Geometry: final body of the model. Coordinates: model frame, mm. Face numbers are marked on the shaded views. A direction names the side the tool comes from. Give positions to 0.01 mm unless a question says otherwise; leave off trailing zeros. Write each loop counter-clockwise with the first axis right and the second up, starting at its lowest first coordinate (ties: lowest second). Pieces come first, ordered by that corner, then holes. Notation, with made-up numbers: (49, -35) -> (62, -35) arc R27 cw to (62, 4) -> close; hole circle Ø10 at (24, -2.75). An arc over 180 degrees is marked (long way). Use CSV: the item, a comma, the result in double quotes. Start each with the question number.
1) Material intervals for line 1 (Z direction, x = 0, y = 8); line 2 (X direction, y = -23, z = -2); line 3 (Y direction, x = -23, z = -13), sorted ascending. Write a range as [from, to].
2) Section A-A (y = 4.5). Output: boundary loops of the cut face in (x, z) (3 decimals).
3) Section C-C (y = -8). Output: boundary loops of the cut face in (x, z).
4) Draft query along X for the marked faces 4, 5 and 6. Return one class per face: pulls with the +X half, pulls with the -X half, needs draft (parallel to the pull), parting line crosses it, or undercut.
5) Contact query for flat-ended pins moving along their axis: P1, Ø2, axis at x = -16.5, y = 3, coming from the +Z side; P2, Ø3, axis at x = 22, z = 0, coming from the -Y side; P3, Ø1, axis at x = 3.5, y = -11, coming from the +Z side; P4, Ø1.5, axis at y = -19.5, z = 1.5, coming from the -X side. Output: stop coordinate, or through.
6) Section B-B (z = -10.75). Output: boundary loops of the cut face in (x, y), plus the area to 3 significant figures.
7) Set-up query: the marked faces 1, 2 and 3. Return all of +Z, -Z, +X, -X, +Y, -Y with unobstructed straight access to the full face (end or side cutting, diameter ignored); none if empty.
8) Section D-D (y = -3). Output: boundary loops of the cut face in (x, z), plus the area to 3 significant figures.
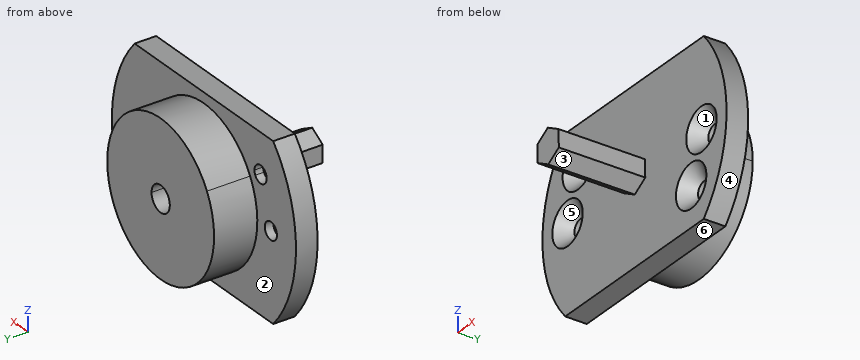
```python
from build123d import *

# Parameters (mm, degrees)
F0_R          = 2
F1_DEPTH      = 5
F2_DEPTH      = 5
F2_DEPTH_BACK = 10
F3_SIZE       = 3
F4_DEPTH      = 25
F5_START      = -2
F5_DEPTH      = 8


with BuildPart() as f1:
    # F0 (on Front) → F1 (new body)
    with BuildSketch(Plane.XZ):
        with BuildLine():
            ThreePointArc((22.7699238258, -19.9146445855), (28.3183041135, -10.6365479426), (30.25, 0))
            ThreePointArc((30.25, 0), (28.3183041135, 10.6365479426), (22.7699238258, 19.9146445855))
            Line((22.7699238258, 19.9146445855), (-22.7699238258, 19.9146445855))
            ThreePointArc((-22.7699238258, 19.9146445855), (-30.25, 0), (-22.7699238258, -19.9146445855))
            Line((-22.7699238258, -19.9146445855), (22.7699238258, -19.9146445855))
        make_face()
        with Locations((18.6195461814, -10.75)):
            Circle(F0_R, mode=Mode.SUBTRACT)
        with Locations((-22, 0)):
            Circle(F0_R, mode=Mode.SUBTRACT)
        with BuildLine():
            ThreePointArc((-16.6195461814, 10.75), (-16.6876945288, 10.2323619098), (-16.8874953738, 9.75))
            ThreePointArc((-16.8874953738, 9.75), (-20.5513978339, 11.2676380902), (-16.6195461814, 10.75))
        make_face(mode=Mode.SUBTRACT)
        with BuildLine():
            ThreePointArc((8.775, 15.1987458364), (15.1987458364, 8.775), (17.55, 0))
            ThreePointArc((17.55, 0), (-4.5422742415, -16.9519982514), (-15.1987458364, 8.775))
            ThreePointArc((-15.1987458364, 8.775), (-4.5422742415, 16.9519982514), (8.775, 15.1987458364))
        make_face(mode=Mode.SUBTRACT)
        with Locations((22, 0)):
            Circle(F0_R, mode=Mode.SUBTRACT)
        with BuildLine():
            ThreePointArc((-15.1987458364, 8.775), (-4.5422742415, -16.9519982514), (17.55, 0))
            ThreePointArc((17.55, 0), (15.1987458364, 8.775), (8.775, 15.1987458364))
            Line((8.775, 15.1987458364), (1.7503574183, 3.0317079799))
            Line((1.7503574183, 3.0317079799), (3.4584509937, 2.0910404247))
            Line((3.4584509937, 2.0910404247), (3.540119625, -1.9495862059))
            Line((3.540119625, -1.9495862059), (0.0816686313, -4.0406266306))
            Line((0.0816686313, -4.0406266306), (-3.4584509937, -2.0910404247))
            Line((-3.4584509937, -2.0910404247), (-3.540119625, 1.9495862059))
            Line((-3.540119625, 1.9495862059), (-3.4603350445, 1.9978253694))
            Line((-3.4603350445, 1.9978253694), (-15.1987458364, 8.775))
        make_face()
        with BuildLine():
            Line((1.7503574183, 3.0317079799), (8.775, 15.1987458364))
            ThreePointArc((8.775, 15.1987458364), (-4.5422742415, 16.9519982514), (-15.1987458364, 8.775))
            Line((-15.1987458364, 8.775), (-3.4603350445, 1.9978253694))
            Line((-3.4603350445, 1.9978253694), (-0.0816686313, 4.0406266306))
            Line((-0.0816686313, 4.0406266306), (1.7503574183, 3.0317079799))
        make_face()
        with BuildLine():
            Line((3.4584509937, 2.0910404247), (1.7503574183, 3.0317079799))
            Line((1.7503574183, 3.0317079799), (1.5, 2.5980762114))
            ThreePointArc((1.5, 2.5980762114), (2.5980762114, 1.5), (3, 0))
            ThreePointArc((3, 0), (-0.7764571353, -2.8977774789), (-2.5980762114, 1.5))
            Line((-2.5980762114, 1.5), (-3.4603350445, 1.9978253694))
            Line((-3.4603350445, 1.9978253694), (-3.540119625, 1.9495862059))
            Line((-3.540119625, 1.9495862059), (-3.4584509937, -2.0910404247))
            Line((-3.4584509937, -2.0910404247), (0.0816686313, -4.0406266306))
            Line((0.0816686313, -4.0406266306), (3.540119625, -1.9495862059))
            Line((3.540119625, -1.9495862059), (3.4584509937, 2.0910404247))
        make_face()
        with BuildLine():
            Line((0, 0), (1.5, 2.5980762114))
            ThreePointArc((1.5, 2.5980762114), (-0.7764571353, 2.8977774789), (-2.5980762114, 1.5))
            Line((-2.5980762114, 1.5), (0, 0))
        make_face()
        with BuildLine():
            Line((1.5, 2.5980762114), (1.7503574183, 3.0317079799))
            Line((1.7503574183, 3.0317079799), (-0.0816686313, 4.0406266306))
            Line((-0.0816686313, 4.0406266306), (-3.4603350445, 1.9978253694))
            Line((-3.4603350445, 1.9978253694), (-2.5980762114, 1.5))
            ThreePointArc((-2.5980762114, 1.5), (-0.7764571353, 2.8977774789), (1.5, 2.5980762114))
        make_face()
        with BuildLine():
            ThreePointArc((3, 0), (2.5980762114, 1.5), (1.5, 2.5980762114))
            Line((1.5, 2.5980762114), (0, 0))
            Line((0, 0), (-2.5980762114, 1.5))
            ThreePointArc((-2.5980762114, 1.5), (-0.7764571353, -2.8977774789), (3, 0))
        make_face()
    extrude(amount=F1_DEPTH)

    # F0 (on Front) → F2 (join, two sides)
    with BuildSketch(Plane.XZ) as f2_sk:
        with BuildLine():
            Line((0, 0), (1.5, 2.5980762114))
            ThreePointArc((1.5, 2.5980762114), (-0.7764571353, 2.8977774789), (-2.5980762114, 1.5))
            Line((-2.5980762114, 1.5), (0, 0))
        make_face()
        with BuildLine():
            ThreePointArc((3, 0), (2.5980762114, 1.5), (1.5, 2.5980762114))
            Line((1.5, 2.5980762114), (0, 0))
            Line((0, 0), (-2.5980762114, 1.5))
            ThreePointArc((-2.5980762114, 1.5), (-0.7764571353, -2.8977774789), (3, 0))
        make_face()
        with BuildLine():
            Line((3.4584509937, 2.0910404247), (1.7503574183, 3.0317079799))
            Line((1.7503574183, 3.0317079799), (1.5, 2.5980762114))
            ThreePointArc((1.5, 2.5980762114), (2.5980762114, 1.5), (3, 0))
            ThreePointArc((3, 0), (-0.7764571353, -2.8977774789), (-2.5980762114, 1.5))
            Line((-2.5980762114, 1.5), (-3.4603350445, 1.9978253694))
            Line((-3.4603350445, 1.9978253694), (-3.540119625, 1.9495862059))
            Line((-3.540119625, 1.9495862059), (-3.4584509937, -2.0910404247))
            Line((-3.4584509937, -2.0910404247), (0.0816686313, -4.0406266306))
            Line((0.0816686313, -4.0406266306), (3.540119625, -1.9495862059))
            Line((3.540119625, -1.9495862059), (3.4584509937, 2.0910404247))
        make_face()
        with BuildLine():
            Line((1.5, 2.5980762114), (1.7503574183, 3.0317079799))
            Line((1.7503574183, 3.0317079799), (-0.0816686313, 4.0406266306))
            Line((-0.0816686313, 4.0406266306), (-3.4603350445, 1.9978253694))
            Line((-3.4603350445, 1.9978253694), (-2.5980762114, 1.5))
            ThreePointArc((-2.5980762114, 1.5), (-0.7764571353, 2.8977774789), (1.5, 2.5980762114))
        make_face()
        with BuildLine():
            ThreePointArc((-15.1987458364, 8.775), (-4.5422742415, -16.9519982514), (17.55, 0))
            ThreePointArc((17.55, 0), (15.1987458364, 8.775), (8.775, 15.1987458364))
            Line((8.775, 15.1987458364), (1.7503574183, 3.0317079799))
            Line((1.7503574183, 3.0317079799), (3.4584509937, 2.0910404247))
            Line((3.4584509937, 2.0910404247), (3.540119625, -1.9495862059))
            Line((3.540119625, -1.9495862059), (0.0816686313, -4.0406266306))
            Line((0.0816686313, -4.0406266306), (-3.4584509937, -2.0910404247))
            Line((-3.4584509937, -2.0910404247), (-3.540119625, 1.9495862059))
            Line((-3.540119625, 1.9495862059), (-3.4603350445, 1.9978253694))
            Line((-3.4603350445, 1.9978253694), (-15.1987458364, 8.775))
        make_face()
        with BuildLine():
            Line((1.7503574183, 3.0317079799), (8.775, 15.1987458364))
            ThreePointArc((8.775, 15.1987458364), (-4.5422742415, 16.9519982514), (-15.1987458364, 8.775))
            Line((-15.1987458364, 8.775), (-3.4603350445, 1.9978253694))
            Line((-3.4603350445, 1.9978253694), (-0.0816686313, 4.0406266306))
            Line((-0.0816686313, 4.0406266306), (1.7503574183, 3.0317079799))
        make_face()
    extrude(amount=F2_DEPTH)
    extrude(f2_sk.sketch, amount=-F2_DEPTH_BACK)

    # F3
    f3_edges = [f1.edges().sort_by_distance(p)[0] for p in [
        (-20.619546, -5, 10.75),
        (16.619546, -5, -10.75),
        (20, -5, 0),
        (-24, -5, 0),
    ]]
    chamfer(f3_edges, length=F3_SIZE)

    # F0 (on Front) → F4 (join)
    with BuildSketch(Plane.XZ):
        with BuildLine():
            Line((1.5, 2.5980762114), (1.7503574183, 3.0317079799))
            Line((1.7503574183, 3.0317079799), (-0.0816686313, 4.0406266306))
            Line((-0.0816686313, 4.0406266306), (-3.4603350445, 1.9978253694))
            Line((-3.4603350445, 1.9978253694), (-2.5980762114, 1.5))
            ThreePointArc((-2.5980762114, 1.5), (-0.7764571353, 2.8977774789), (1.5, 2.5980762114))
        make_face()
        with BuildLine():
            Line((3.4584509937, 2.0910404247), (1.7503574183, 3.0317079799))
            Line((1.7503574183, 3.0317079799), (1.5, 2.5980762114))
            ThreePointArc((1.5, 2.5980762114), (2.5980762114, 1.5), (3, 0))
            ThreePointArc((3, 0), (-0.7764571353, -2.8977774789), (-2.5980762114, 1.5))
            Line((-2.5980762114, 1.5), (-3.4603350445, 1.9978253694))
            Line((-3.4603350445, 1.9978253694), (-3.540119625, 1.9495862059))
            Line((-3.540119625, 1.9495862059), (-3.4584509937, -2.0910404247))
            Line((-3.4584509937, -2.0910404247), (0.0816686313, -4.0406266306))
            Line((0.0816686313, -4.0406266306), (3.540119625, -1.9495862059))
            Line((3.540119625, -1.9495862059), (3.4584509937, 2.0910404247))
        make_face()
        with BuildLine():
            ThreePointArc((3, 0), (2.5980762114, 1.5), (1.5, 2.5980762114))
            Line((1.5, 2.5980762114), (0, 0))
            Line((0, 0), (-2.5980762114, 1.5))
            ThreePointArc((-2.5980762114, 1.5), (-0.7764571353, -2.8977774789), (3, 0))
        make_face()
        with BuildLine():
            Line((0, 0), (1.5, 2.5980762114))
            ThreePointArc((1.5, 2.5980762114), (-0.7764571353, 2.8977774789), (-2.5980762114, 1.5))
            Line((-2.5980762114, 1.5), (0, 0))
        make_face()
    extrude(amount=F4_DEPTH)

    # F0 (on Front) → F5 (cut)
    with BuildSketch(Plane.XZ.offset(F5_START)):
        with BuildLine():
            ThreePointArc((3, 0), (2.5980762114, 1.5), (1.5, 2.5980762114))
            Line((1.5, 2.5980762114), (0, 0))
            Line((0, 0), (-2.5980762114, 1.5))
            ThreePointArc((-2.5980762114, 1.5), (-0.7764571353, -2.8977774789), (3, 0))
        make_face()
        with BuildLine():
            Line((0, 0), (1.5, 2.5980762114))
            ThreePointArc((1.5, 2.5980762114), (-0.7764571353, 2.8977774789), (-2.5980762114, 1.5))
            Line((-2.5980762114, 1.5), (0, 0))
        make_face()
    extrude(amount=-F5_DEPTH, mode=Mode.SUBTRACT)


solid = f1.part
```
Answers follow:
1,line 1,"z = [-17.55, -3], [3, 17.55]"
1,line 2,"x = [-3.46, 3.46]"
1,line 3,"y = [-5, 0]"
2,outline,"circle Ø35.1 at (0, 0); hole circle Ø6 at (0, 0)"
3,outline,"(-3.54, 1.95) -> (-3.46, -2.09) -> (0.08, -4.04) -> (3.54, -1.95) -> (3.46, 2.09) -> (-0.08, 4.04) -> close"
4,face 4,"pulls with the +X half"
4,face 5,"undercut"
4,face 6,"needs draft"
5,P1,"stops at z = 8.23"
5,P2,"passes through"
5,P3,"stops at z = 2.34"
5,P4,"stops at x = -3.54"
6,outline,"(-28.28, -5) -> (13.62, -5) -> (16.62, -2) -> (16.62, 0) -> (13.87, 0) -> (13.87, 10) -> (-13.87, 10) -> (-13.87, 0) -> (-28.28, 0) -> close; (20.62, -2) -> (23.62, -5) -> (28.28, -5) -> (28.28, 0) -> (20.62, 0) -> close"
6,area,"531 mm^2"
7,face 1,"-Y"
7,face 2,"+Y"
7,face 3,"-Z, +X, -Y"
8,outline,"(-22.77, -19.91) -> (22.77, -19.91) arc R30.25 ccw to (22.77, 19.91) -> (-22.77, 19.91) arc R30.25 ccw to start; hole circle Ø6 at (-22, 0); hole circle Ø6 at (-18.62, 10.75); hole circle Ø6 at (18.62, -10.75); hole circle Ø6 at (22, 0)"
8,area,"2,110 mm^2"
